Autodesk Inventor part; units mm, degrees
ref_plane "YZ Plane" through (0, 0, 0) normal (1, 0, 0) x (0, 1, 0)
ref_plane "XZ Plane" through (0, 0, 0) normal (0, 1, 0) x (-1, 0, 0)
ref_plane "XY Plane" through (0, 0, 0) normal (0, 0, 1) x (1, 0, 0)
sketch "Sketch1" plane through (0, 0, 0) normal (0, 1, 0) x (-1, 0, 0)
  circle A0 centre (0, 0) radius 5.5
  dimension "d0" = 11
extrude "Extrusion1" add sketch "Sketch1" along normal blind 38
sketch "Sketch6" plane through (0, 0, 0) normal (0, -1, 0) x (1, 0, 0)
  circle A0 centre (0, 0) radius 5.5
  line L0 (3.45, 0) -> (3.45, -4.2834)
  line L1 (0.45, 0) -> (0.45, -5.4816)
  line L2 (3.45, -5.4816) -> (3.45, -4.2834)
  line L3 (3.45, -5.4816) -> (0.45, -5.4816)
  line L4 (0.45, 0) -> (0.45, 5.4816)
  line L5 (3.45, 5.3243) -> (3.45, 0)
  line L6 (3.45, 5.3243) -> (0.45, 5.4816)
  line L7 (0, -5.5) -> (0, 5.5)
  line L8 (-3.45, 0) -> (-3.45, -4.2834)
  line L9 (-0.45, 0) -> (-0.45, -5.4816)
  line L10 (-3.45, -5.4816) -> (-3.45, -4.2834)
  line L11 (-3.45, -5.4816) -> (-0.45, -5.4816)
  line L12 (-0.45, 0) -> (-0.45, 5.4816)
  line L13 (-3.45, 5.3243) -> (-3.45, 0)
  line L14 (-3.45, 5.3243) -> (-0.45, 5.4816)
  point P0 (-3.45, 4.2834)
  point P1 (3.45, 4.2834)
  dimension "d20" = 3
  dimension "d21" = 3
  dimension "d22" = 0.45
  dimension "d23" = 2.05
  dimension "d24" = 2.05
extrude "Extrusion5" add sketch "Sketch6" along normal blind 6 contours A0 L5 L0 L1 L4 | L12 L9 A0 L8 L13
sketch "Sketch8" plane through (0, 0, 0) normal (1, 0, 0) x (0, 1, 0)
  line L0 (0, -5.5) -> (38, -5.5)
  line L1 (0, -5.4816) -> (-6, -5.4816)
  line L2 (0, -5.4816) -> (0, 5.4816)
  line L3 (0, -5.4816) -> (-6, 0.5184)
  line L4 (0, -5.4816) -> (8.4853, -5.4816) construction
  line L5 (-6, -5.4816) -> (-6, 5.4816)
  line L6 (-6, 0.5184) -> (-6, -5.4816)
  point P0 (0, 0)
  dimension "d27" = 135
extrude "Extrusion6" cut sketch "Sketch8" along normal through all both and the other way through all
sketch "Sketch10" plane through (0, 0, 0) normal (1, 0, 0) x (0, 1, 0)
  circle A0 centre (-3.5, 0) radius 1
  line L0 (0, -5.5) -> (38, -5.5)
  line L1 (-6, 0.5184) -> (-6, 5.4816)
  point P0 (0, 0)
  dimension "d30" = 2
  dimension "d31" = 5.5
  dimension "d32" = 2.5
extrude "Extrusion7" cut sketch "Sketch10" along normal through all both and the other way through all
sketch "Sketch11" plane through (0, 38, 0) normal (0, 1, 0) x (1, 0, 0)
  circle A0 centre (0, 2.5) radius 1
  circle A1 centre (0, -2.5) radius 1
  point P0 (0, 0)
  dimension "d35" = 2
  dimension "d36" = 2
  dimension "d37" = 2.5
  dimension "d38" = 2.5
extrude "Extrusion8" cut sketch "Sketch11" against normal blind 38
properties part number "Part4 finger(index)"
Geometry: final body of the model. Coordinates: model frame, mm. A direction names the side the tool comes from. Round coordinates to 2 decimals unless told otherwise and drop trailing zeros. Loops run counter-clockwise (first coordinate to the right, second up) from the corner with the lowest first, then second, coordinate; pieces in that order, holes last.
Q1. Pull-direction query (X, two-part tool) for faces 1 (the flat face through (-0.45, -2, 1)), 2 (the flat face through (4, 0, 0)), 3 (the cylindrical face through (1.19, 15.69, 5.37)); classes: released by +X, released by -X, zero draft, split by the parting line, or undercut.
Q2. Pin query (flat end, axial travel): P1, Ø1.6, axis at x = -4.5, z = 2, coming from the -Y side; P2, Ø3, axis at y = 32, z = 1.5, coming from the -X side; P3, Ø1.8, axis at y = -3.5, z = 0, coming from the -X side; P4, Ø3, axis at y = -2, z = 2, coming from the -X side. Return the tip coordinate at first contact, or that it passes through.
Q3. Section A-A on z = 0. Return loops of the section in (x, y).
Q4. Access query for faces 4 (the flat face through (0, 0, 4)), 5 (the flat face through (3.45, -2, 1)), 6 (the flat face through (-4, 0, 0)), 7 (the cylindrical face through (-0.217, 19.266, 3.476)). Directions: +Z, -Z, +X, -X, +Y, -Y. A direction counts if a zero-diameter tool reaches every point of the face in a straight line with its end or side. Return the directions, or none.
Q5. Section B-B on z = 2.5. Return loops of the section in (x, y).
Q6. Section C-C on y = -3.5. Return loops of the section in (x, z).
Q7. Section D-D on x = 1.75. Return loops of the section in (y, z).
Q8. Material intervals for L1, parallel to Z at x = 0, y = 21; L2, parallel to X at y = -2, z = -0.25; L3, parallel to Z at x = -0.5, y = 22, sorted ascending.
Evaluation:
1. face 1: undercut
1. face 2: zero draft
1. face 3: split by the parting line
2. P1: stops at y = 0
2. P2: stops at x = -5.5
2. P3: passes through
2. P4: stops at x = -3.45
3. outline: (-5.5, 0) - (-3.45, 0) - (-3.45, -2.5) - (-0.45, -2.5) - (-0.45, 0) - (0.45, 0) - (0.45, -2.5) - (3.45, -2.5) - (3.45, 0) - (5.5, 0) - (5.5, 38) - (-5.5, 38) - close; (-3.45, -5.48) - (-0.45, -5.48) - (-0.45, -4.5) - (-3.45, -4.5) - close; (0.45, -5.48) - (3.45, -5.48) - (3.45, -4.5) - (0.45, -4.5) - close
4. face 4: +Z, -Z, -Y
4. face 5: +Z, -Z, +X, -Y
4. face 6: +Z, -Z, -X, -Y
4. face 7: +Y
5. outline: (-4.9, 0) - (-3.45, 0) - (-3.45, -6) - (-0.45, -6) - (-0.45, 0) - (-1, 0) - (-1, 38) - (-4.9, 38) - close; (0.45, -6) - (3.45, -6) - (3.45, 0) - (4.9, 0) - (4.9, 38) - (1, 38) - (1, 0) - (0.45, 0) - close
6. outline: (-3.45, -1.98) - (-0.45, -1.98) - (-0.45, -1) - (-3.45, -1) - close; (-3.45, 1) - (-0.45, 1) - (-0.45, 5.48) arc R5.5 ccw to (-3.45, 4.28) - close; (0.45, -1.98) - (3.45, -1.98) - (3.45, -1) - (0.45, -1) - close; (0.45, 1) - (3.45, 1) - (3.45, 4.28) arc R5.5 ccw to (0.45, 5.48) - close
7. outline: (-6, 0.52) - (-0.27, -5.21) - (38, -5.21) - (38, 5.21) - (-6, 5.21) - close; hole circle Ø2 at (-3.5, 0)
8. L1: z = -5.5 to -3.5, -1.5 to 1.5, 3.5 to 5.5
8. L2: x = -3.45 to -0.45, 0.45 to 3.45
8. L3: z = -5.48 to -3.37, -1.63 to 1.63, 3.37 to 5.48
